Source: three-view drawing plus pictorial views. Frame: mm from the lowest corner of the part. Coordinates: 2 decimals unless noted, no trailing zeros. Write each loop counter-clockwise with the first axis right and the second up, starting at its lowest first coordinate (ties: lowest second). Pieces come first, ordered by that corner, then holes. Notation, with made-up numbers: (48.25, 55) - (100.25, 55) arc R15 ccw to (100.25, 83) - close; hole circle Ø3 at (8, 55). An arc over 180 degrees is marked (long way). Answer as a JSON object with one key per item and string values. Group by question number.
Item 1: First-contact query: pin 1 Ø20 at (x, y) = (23, 31.5) entering from +Z; pin 2 Ø0.8 at (x, z) = (23.5, 3.5) entering from -Y; pin 3 Ø1 at (x, y) = (10, 32) entering from -Z; pin 4 Ø2.5 at (x, z) = (22.5, 5) entering from -Y. Flat tips, straight axial feed; report the tip coordinate or a pass-through.
Item 2: Section A-A on y = 8. Return loops of the section in (x, z) (3 decimals), and give its area (3 significant figures).
Item 3: Line query: line 1 along Y through (x, z) = (20, 0.5); line 2 along Z through (x, y) = (33, 7); line 3 along Y through (x, z) = (19, 1.5). Output: solid intervals per line, ascending. Write a range as from..to.
Item 4: Section B-B on x = 15. Return loops of the section in (y, z).
Item 5: Section C-C on z = 5. Return loops of the section in (x, y).
Item 6: Section D-D on y = 33. Return loops of the section in (x, z), and give its area (3 significant figures).
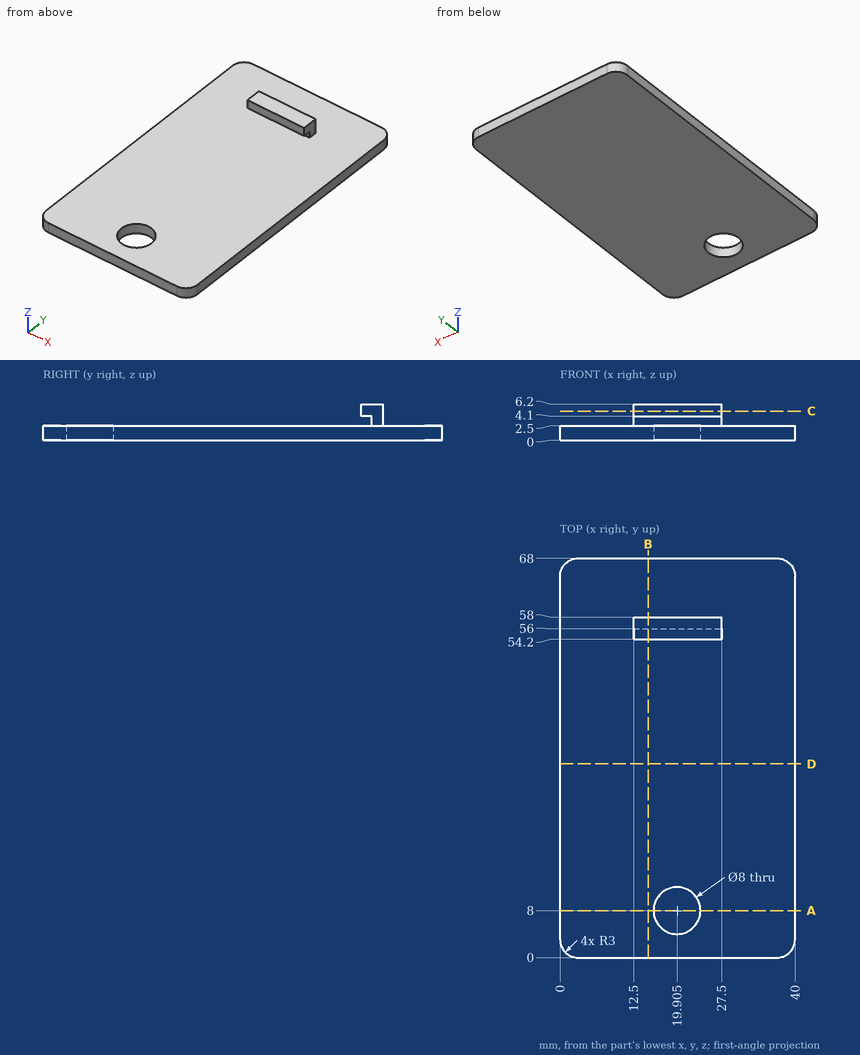
Checks:
{
 "1": {"pin 1": "z = 2.5", "pin 2": "y = 56", "pin 3": "z = 0", "pin 4": "y = 54.2"},
 "2": {"outline": "(0, 0) - (15.905, 0) - (15.905, 2.5) - (0, 2.5) - close; (23.905, 0) - (40, 0) - (40, 2.5) - (23.905, 2.5) - close", "area": "80.0 mm^2"},
 "3": {"line 1": "0..4, 12..68", "line 2": "0..2.5", "line 3": "0..4.1, 11.9..68"},
 "4": {"outline": "(0, 0) - (68, 0) - (68, 2.5) - (58, 2.5) - (58, 6.2) - (54.2, 6.2) - (54.2, 4.1) - (56, 4.1) - (56, 2.5) - (0, 2.5) - close"},
 "5": {"outline": "(12.5, 54.2) - (27.5, 54.2) - (27.5, 58) - (12.5, 58) - close"},
 "6": {"outline": "(0, 0) - (40, 0) - (40, 2.5) - (0, 2.5) - close", "area": "100 mm^2"}
}
